Input: dimensioned drawing with shaded views. Units: mm. Origin: part minimum x, y, z. Coordinates: 2 decimals unless noted, no trailing zeros. Loops run counter-clockwise (first coordinate to the right, second up) from the corner with the lowest first, then second, coordinate; pieces in that order, holes last. Notation, with made-up numbers: (-2.75, 2.25) - (37.25, 2.25) arc R33 ccw to (37.25, 41.25) - close; hole circle Ø8 at (-20.75, 32.5). An arc over 180 degrees is marked (long way). Put each result on its own line as item: value. Start each with the question number.
1) Section C-C on x = 2.4. Count the separate pieces of the cut face and the enclosed holes in it, and give its area (3 significant figures).
2) Section D-D on y = 125. Output: boundary loops of the cut face in (x, z) (3 decimals), and give its area (3 significant figures).
3) Material intervals for line 1 along Z through (x, y) = (1.05, 25.4); line 2 along Z through (x, y) = (2.4, 165.1); line 3 along Y through (x, z) = (1.65, 31), sorted ascending. Write a range as from..to.
4) Section B-B on y = 31. Output: boundary loops of the cut face in (x, z) (3 decimals).
5) Contact query for flat-ended pins moving along their axis: pin 1 Ø23 at (y, z) = (165.1, 25.4) entering from -X; pin 2 Ø1.6 at (x, y) = (2, 107) entering from +Z. Output: stop coordinate, or through.
6) Section A-A on z = 25.4. Output: boundary loops of the cut face in (x, y) (1 decimal).
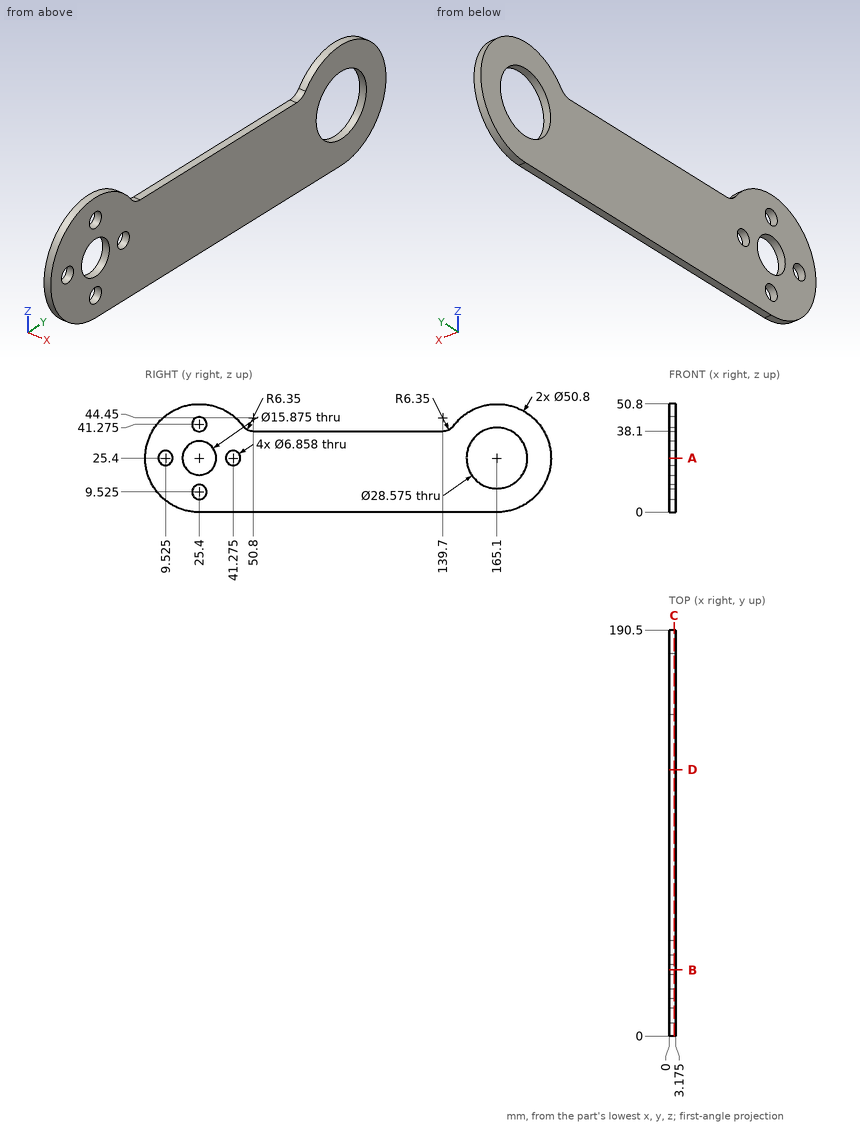
Answer block:
1. separate pieces: 1
1. enclosed holes: 6
1. area: 6,760 mm²
2. outline: (0, 0) - (3.175, 0) - (3.175, 38.1) - (0, 38.1) - close
2. area: 121 mm²
3. line 1: z = 0..6.1, 12.95..17.46, 33.34..37.85, 44.7..50.8
3. line 2: z = 0..11.11, 39.69..50.8
3. line 3: y = 0.63..19.77, 31.03..151.96, 178.24..189.87
4. outline: (0, 0) - (3.175, 0) - (3.175, 19.775) - (0, 19.775) - close; (0, 31.025) - (3.175, 31.025) - (3.175, 50.175) - (0, 50.175) - close
5. pin 1: passes through
5. pin 2: stops at z = 38.1
6. outline: (0, 0) - (3.2, 0) - (3.2, 6.1) - (0, 6.1) - close; (0, 13) - (3.2, 13) - (3.2, 17.5) - (0, 17.5) - close; (0, 33.3) - (3.2, 33.3) - (3.2, 37.8) - (0, 37.8) - close; (0, 44.7) - (3.2, 44.7) - (3.2, 150.8) - (0, 150.8) - close; (0, 179.4) - (3.2, 179.4) - (3.2, 190.5) - (0, 190.5) - close
